Can you work these out from the drawing? Everything is in mm from the part's minimum corner. A direction names the side the tool comes from. Coordinates: 2 decimals unless noted, no trailing zeros. Loops run counter-clockwise (first coordinate to the right, second up) from the corner with the lowest first, then second, coordinate; pieces in that order, holes last. Notation, with made-up numbers: (78, 4) - (132, 4) arc R25 cw to (132, 20) - close; hole circle Ø3 at (83, 71). An arc over 180 degrees is marked (long way). One line per question, with ' | ' between items. Start each with the question number.
1. Please list where these lines run through material, in increasing order: L1, parallel to Z at x = 15, y = 10.25; L2, parallel to Z at x = 25.25, y = 13.5; L3, parallel to X at y = 4.25, z = 35. Write a range as [from, to].
2. I want a section at D-D, the plane x = 15.5. Write out the boundary of the cut face in (y, z).
3. We'd pull the mould along Z, two halves only. Please class the marked faces 3, 4, 5 and 6: pulls with the +Z half, pulls with the -Z half, needs draft (parallel to the pull), parting line crosses it, or undercut.
4. I'm going to push flat-ended pins straight in: P1, Ø9, axis at y = 6, z = 16.5, coming from the -X side; P2, Ø1.8, axis at x = 15, z = 2, coming from the -Y side. Where does each tip first touch, or does it pass through?
5. I want a section at B-B, the plane z = 13. Write out the boundary of the cut face in (x, y).
6. I want a section at A-A, the plane y = 13.25. Write out the boundary of the cut face in (x, z).
7. Which directions (+Z, -Z, +X, -X, +Y, -Y) give clear straight access to the entire face, cutting with the end or side of a thin tool? Please do the marked faces 1 and 2.
8. I want a section at C-C, the plane x = 21. Write out the boundary of the cut face in (y, z).
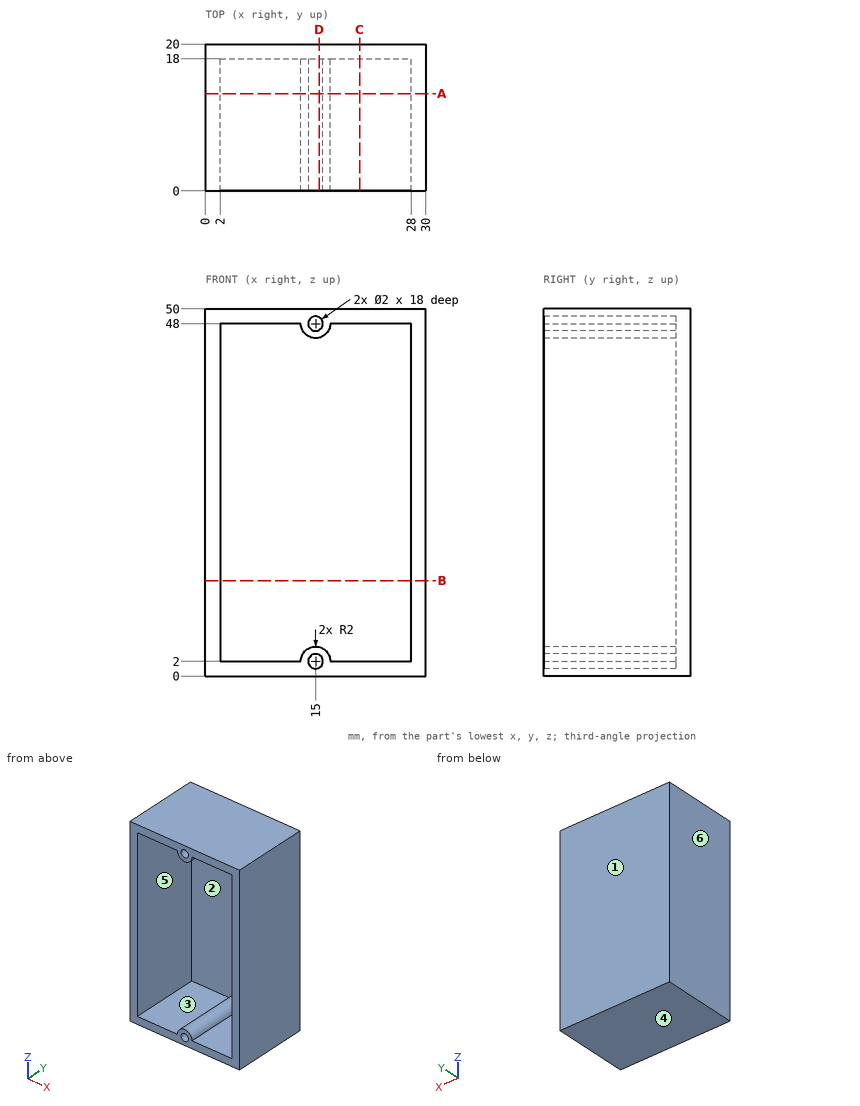
Results are:
1) L1: z = [0, 1], [3, 4], [46, 47], [49, 50] | L2: z = [0, 2], [48, 50] | L3: x = [0, 2], [28, 30]
2) outline: (0, 0) - (20, 0) - (20, 50) - (0, 50) - (0, 48.87) - (18, 48.87) - (18, 47.13) - (0, 47.13) - (0, 46.06) - (18, 46.06) - (18, 3.94) - (0, 3.94) - (0, 2.87) - (18, 2.87) - (18, 1.13) - (0, 1.13) - close
3) face 3: undercut | face 4: pulls with the -Z half | face 5: undercut | face 6: needs draft
4) P1: stops at x = 0 | P2: stops at y = 18
5) outline: (0, 0) - (2, 0) - (2, 18) - (28, 18) - (28, 0) - (30, 0) - (30, 20) - (0, 20) - close
6) outline: (0, 0) - (30, 0) - (30, 50) - (0, 50) - close; hole (2, 2) - (13, 2) arc R2 cw to (17, 2) - (28, 2) - (28, 48) - (17, 48) arc R2 cw to (13, 48) - (2, 48) - close; hole circle Ø2 at (15, 2); hole circle Ø2 at (15, 48)
7) face 1: +Z, -Z, +X, -X, +Y | face 2: -Y
8) outline: (0, 0) - (20, 0) - (20, 50) - (0, 50) - (0, 48) - (18, 48) - (18, 2) - (0, 2) - close
